CAD build for the part. Positions are in the model's coordinates, mm. Face numbers are marked on the shaded views. A direction names the side the tool comes from. Coordinates: 2 decimals unless noted, no trailing zeros. Order: outer loops, then holes, each group sorted by start corner. A loop starts at its lowest first (then second) coordinate and runs counter-clockwise, first axis right, second up. Notation, with made-up numbers: M 39.5,13 L 43.5,13 A21 cw 43.5,42 Z; hole C 47.5,34.5 d8. An arc over 180 degrees is marked long. Write item = value, one per line. Start each with the question number.
```python
from build123d import *

# Parameters (mm, degrees)
BOSS_EXTRUDE2_DEPTH = 15
FILLET5_R           = 15
FILLET6_R           = 15
FILLET7_R           = 15
FILLET8_R           = 15
SKETCH4_R           = 2.05
CUT_EXTRUDE2_DEPTH  = 23


with BuildPart() as part:
    # Sketch3 → Boss-Extrude2 (new body)
    with BuildSketch(Plane.XY):
        with BuildLine():
            Line((-1.5, 40), (-1.5, 15.979752814))
            ThreePointArc((-1.5, 15.979752814), (0, -16.05), (1.5, 15.979752814))
            Line((1.5, 15.979752814), (1.5, 30))
            Line((1.5, 30), (1.5, 40))
            Line((1.5, 40), (11.5, 40))
            Line((11.5, 40), (11.5, 30))
            Line((11.5, 30), (30, 30))
            Line((30, 30), (30, -30))
            Line((30, -30), (-30, -30))
            Line((-30, -30), (-30, 30))
            Line((-30, 30), (-11.5, 30))
            Line((-11.5, 30), (-11.5, 40))
            Line((-11.5, 40), (-1.5, 40))
        make_face()
    extrude(amount=BOSS_EXTRUDE2_DEPTH)

    # Fillet5
    fillet5_edges = [part.edges().sort_by_distance(p)[0] for p in [
        (30, 30, 7.5),
    ]]
    fillet(fillet5_edges, radius=FILLET5_R)

    # Fillet6
    fillet6_edges = [part.edges().sort_by_distance(p)[0] for p in [
        (-30, 30, 7.5),
    ]]
    fillet(fillet6_edges, radius=FILLET6_R)

    # Fillet7
    fillet7_edges = [part.edges().sort_by_distance(p)[0] for p in [
        (-30, -30, 7.5),
    ]]
    fillet(fillet7_edges, radius=FILLET7_R)

    # Fillet8
    fillet8_edges = [part.edges().sort_by_distance(p)[0] for p in [
        (30, -30, 7.5),
    ]]
    fillet(fillet8_edges, radius=FILLET8_R)

    # Sketch4 → Cut-Extrude2 (cut)
    with BuildSketch(Plane(origin=(11.5, 0, 0), x_dir=(0, 0, -1), z_dir=(1, 0, 0))):
        with Locations((-7.5, 35)):
            Circle(SKETCH4_R)
    extrude(amount=-CUT_EXTRUDE2_DEPTH, mode=Mode.SUBTRACT)


solid = part.part
```
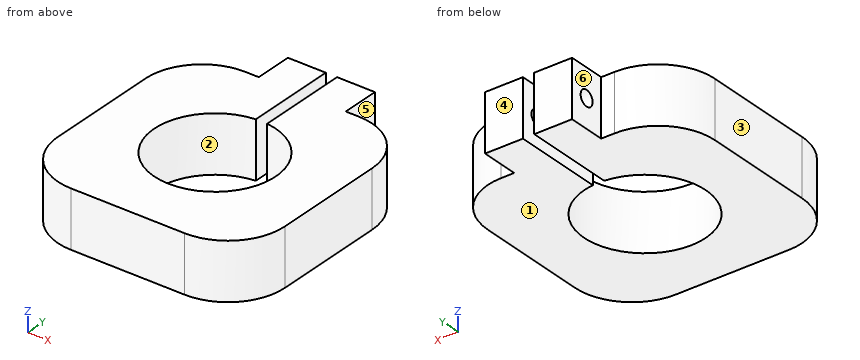
1. Slice it at B-B (y = 35). Write the cut outline in (x, z), plus the area to 3 significant figures.
2. Probe L1, parallel to Y at x = -3.25, z = 7.5; L2, parallel to Y at x = 7.5, z = 7; L3, parallel to X at y = 34, z = 1.25. List the from-to ranges inside material, lowest first.
3. Flat gauge pins, fed straight in: pin 1 (1.1 mm diameter, centred on x = -14, z = 5.5, fed in from +Y); pin 2 (3.5 mm diameter, centred on y = 35, z = 7.5, fed in from -X); pin 3 (4.5 mm diameter, centred on y = 35, z = 7.5, fed in from -X); pin 4 (5 mm diameter, centred on y = 34, z = 4.5, fed in from +X). Where does each tip first touch, or does it go through?
4. Slice it at C-C (x = -3.5). Write the cut outline in (y, z), plus the area to 3 significant figures.
5. Slice it at D-D (y = 21). Write the cut outline in (x, z).
6. 3-axis set-ups, long thin cutter, end or side, ignore diameter. For the marked faces 4, 5 and 6: which of +Z, -Z, +X, -X, +Y, -Y reach the whole face in a straight line?
7. Slice it at A-A (z = 7.5). Write the cut outline in (x, y), plus the area to 3 significant figures.
8. Mould opens along X. For the marked faces 1, 2 and 3 say: released by +X, released by -X, zero draft, split by the parting line, or undercut.
Calculated:
q1.outline = M -11.5,0 L -1.5,0 L -1.5,5.45 L -11.5,5.45 Z; M -11.5,9.55 L -1.5,9.55 L -1.5,15 L -11.5,15 Z; M 1.5,0 L 11.5,0 L 11.5,5.45 L 1.5,5.45 Z; M 1.5,9.55 L 11.5,9.55 L 11.5,15 L 1.5,15 Z
q1.area = 218 mm²
q2.L1 = -30 to -15.72, 15.72 to 32.95, 37.05 to 40
q2.L2 = -30 to -14.19, 14.19 to 33.01, 36.99 to 40
q2.L3 = -11.5 to -1.5, 1.5 to 11.5
q3.pin_1 = 30
q3.pin_2 = through
q3.pin_3 = -11.5
q3.pin_4 = 11.5
q4.outline = M -30,0 L -15.66,0 L -15.66,15 L -30,15 Z; M 15.66,0 L 40,0 L 40,15 L 15.66,15 Z; hole C 35,7.5 d4.1
q4.area = 567 mm²
q5.outline = M -28.75,0 L -1.5,0 L -1.5,15 L -28.75,15 Z; M 1.5,0 L 28.75,0 L 28.75,15 L 1.5,15 Z
q6.face_4 = +Z, -Z, +X, -X, +Y
q6.face_5 = +Z, -Z, +X, +Y
q6.face_6 = +Z, -Z, -X, +Y
q7.outline = M -30,-15 A15 ccw -15,-30 L 15,-30 A15 ccw 30,-15 L 30,15 A15 ccw 15,30 L 11.5,30 L 11.5,32.95 L 1.5,32.95 L 1.5,15.98 A16.05 cw long -1.5,15.98 L -1.5,32.95 L -11.5,32.95 L -11.5,30 L -15,30 A15 ccw -30,15 Z; M -11.5,37.05 L -1.5,37.05 L -1.5,40 L -11.5,40 Z; M 1.5,37.05 L 11.5,37.05 L 11.5,40 L 1.5,40 Z
q7.area = 2,670 mm²
q8.face_1 = zero draft
q8.face_2 = undercut
q8.face_3 = released by -X
